The model under review builds one solid part; all positions refer to its coordinate system, in mm. Give positions to 0.01 mm unless a question says otherwise; leave off trailing zeros. Order: outer loops, then holes, each group sorted by start corner. A loop starts at its lowest first (then second) coordinate and runs counter-clockwise, first axis right, second up. Notation, with made-up numbers: (-31, -15.75) - (9, -15.75) arc R6 cw to (9, -11.75) - close; hole circle Ø7 at (-20, 5). An arc over 180 degrees is marked (long way). Use a Markdown table: item, result. Add a question column.
```python
from build123d import *

# Parameters (mm, degrees)
BOSS_EXTRUDE1_DEPTH                = 6
TAP_DRILL_FOR_M2_5X0_45_TAP1_D     = 2.05
TAP_DRILL_FOR_M2_5X0_45_TAP1_DEPTH = 19


with BuildPart() as part:
    # Sketch1 → Boss-Extrude1 (new body)
    with BuildSketch(Plane(origin=(0, 6, 0), x_dir=(1, 0, 0), z_dir=(0, 1, 0))):
        Polygon((1.356773133, -2.35), (2.713546265, 0), (1.356773133, 2.35), (-1.356773133, 2.35), (-2.713546265, 0), (-1.356773133, -2.35), align=None)
    extrude(amount=-BOSS_EXTRUDE1_DEPTH)

    # Tap Drill for M2.5x0.45 Tap1
    with Locations(Plane(origin=(0, 6, 0), x_dir=(1, 0, 0), z_dir=(0, 1, 0))):
        with Locations((0, 0)):
            Hole(TAP_DRILL_FOR_M2_5X0_45_TAP1_D / 2, depth=TAP_DRILL_FOR_M2_5X0_45_TAP1_DEPTH)


solid = part.part
```
Q1. We need section B-B (x = 0). Write out the cut boundary in (y, z) (3 decimals), plus the area to 3 significant figures.
Q2. Draft analysis for pull direction Z (two halves, no side actions). For faces 1 (the flat face through (2.026, 3.042, 1.191)), 2 (the flat face through (0, 3, -2.35)), 3 (the cylindrical face through (0.133, 2.958, -1.016)), state which applies: pulls with the +Z half, pulls with the -Z half, needs draft (parallel to the pull), parting line crosses it, or undercut.
Q3. We need section C-C (z = 0.35). Write out the cut boundary in (x, y).
Q4. We need section A-A (y = 1.85). Write out the cut boundary in (x, z) (3 decimals), plus the area to 3 significant figures.
Q5. We need section D-D (x = -1.65). Write out the cut boundary in (y, z), plus the area to 3 significant figures.
Q6. Wall thickness on probe 1 along Z at (x, y) = (0, 1.8) (3 decimals); probe 2 along X at (y, z) = (0.9, -0.05); probe 3 along X at (y, z) = (5.7, 0.45): over which ranges is each line inside the solid? List them lowest first.
Here are the results:
| question | item | result |
|---|---|---|
| 1 | outline | (0, -2.35) - (6, -2.35) - (6, -1.025) - (0, -1.025) - close; (0, 1.025) - (6, 1.025) - (6, 2.35) - (0, 2.35) - close |
| 1 | area | 15.9 mm2 |
| 2 | face 1 | pulls with the +Z half |
| 2 | face 2 | pulls with the -Z half |
| 2 | face 3 | undercut |
| 3 | outline | (-2.51, 0) - (-0.96, 0) - (-0.96, 6) - (-2.51, 6) - close; (0.96, 0) - (2.51, 0) - (2.51, 6) - (0.96, 6) - close |
| 4 | outline | (-2.714, 0) - (-1.357, -2.35) - (1.357, -2.35) - (2.714, 0) - (1.357, 2.35) - (-1.357, 2.35) - close; hole circle Ø2.05 at (0, 0) |
| 4 | area | 15.8 mm2 |
| 5 | outline | (0, -1.84) - (6, -1.84) - (6, 1.84) - (0, 1.84) - close |
| 5 | area | 22.1 mm2 |
| 6 | probe 1 | -2.35 to -1.025, 1.025 to 2.35 |
| 6 | probe 2 | -2.68 to -1.02, 1.02 to 2.68 |
| 6 | probe 3 | -2.45 to -0.92, 0.92 to 2.45 |
